Can you work these out from the model? Positions are in its coordinate system, mm. A direction names the side the tool comes from. Give positions to 0.01 mm unless a question says otherwise; leave off trailing zeros. Loops run counter-clockwise (first coordinate to the right, second up) from the corner with the lowest first, then second, coordinate; pieces in that order, holes last.
Solid Edge part; units mm, degrees
sketch "Sketch1" plane through (0, 0, 0) normal (1, 0, 0) x (0, 1, 0)
  circle A0 centre (0, 0) radius 2.5
extrude "Protrusion1" add sketch "Sketch1" along normal mid plane 40
sketch "Sketch2" plane through (0, 0, 0) normal (0, -1, 0) x (1, 0, 0)
  line L0 (30, 0) -> (30, 20)
  line L1 (30, -10) -> (30, 0)
  line L2 (20, -10) -> (30, -10)
  line L3 (20, 20) -> (20, -10)
  line L4 (20, 20) -> (-20, 20)
  line L5 (-20, -10) -> (-20, 20)
  line L6 (-30, -10) -> (-20, -10)
  line L7 (-30, 0) -> (-30, -10)
  line L8 (-30, 20) -> (-30, 0)
  line L9 (-30, 30) -> (-30, 20)
  line L10 (30, 30) -> (-30, 30)
  line L11 (30, 20) -> (30, 30)
extrude "ExtrudedProtrusion_2" add sketch "Sketch2" along normal mid plane 10
(1) Suppose I cut it at C-C on x = -14. List the corners of the cut face in (y, z) for me, plus the area to 3 significant figures.
Returned:
outline: (-5, 20) - (5, 20) - (5, 30) - (-5, 30) - close; circle Ø5 at (0, 0)
area: 120 mm2
(2) Will these pins go through, and if not, where does the flat tip stop? P1, Ø2, axis at x = -7, z = 18.5, coming from the -Y side; P2, Ø1, axis at x = -3, y = 2, coming from the -Z side.
Returned:
P1: passes through
P2: stops at z = -2
(3) Which directions (+Z, -Z, +X, -X, +Y, -Y) give clear straight access to the entire face, cutting with the end or side of a thin tool? Please do faces 5 (the flat face through (0, 0, 30)), 6 (the flat face through (0, 0, 20)).
Returned:
face 5: +Z, +X, -X, +Y, -Y
face 6: +Y, -Y
(4) Suppose I cut it at A-A on z = 6.5. List the corners of the cut face in (x, y) for me.
Returned:
outline: (-30, -5) - (-20, -5) - (-20, 5) - (-30, 5) - close; (20, -5) - (30, -5) - (30, 5) - (20, 5) - close
(5) Suppose I cut it at D-D on y = -3.75. List the corners of the cut face in (x, z) for me.
Returned:
outline: (-30, -10) - (-20, -10) - (-20, 20) - (20, 20) - (20, -10) - (30, -10) - (30, 30) - (-30, 30) - close
(6) Please list where these lines run through material, in increasing order: probe 1 along X at (y, z) = (0, 13); probe 2 along Z at (x, y) = (18, 0.25); probe 3 along Z at (x, y) = (-16.5, -3).
Returned:
probe 1: x = -30 to -20, 20 to 30
probe 2: z = -2.49 to 2.49, 20 to 30
probe 3: z = 20 to 30
(7) Thinking about a two-plate mould opening in X: for faces 1 (the flat face through (30, 0, 10)), 2 (the cylindrical face through (0.28, -0.54, -2.44)), 3 (the flat face through (-30, 0, 10)), 4 (the flat face through (-25, 0, -10)), which applies, pulls with the +X half, pulls with the -X half, needs draft (parallel to the pull), parting line crosses it, or undercut?
Returned:
face 1: pulls with the +X half
face 2: undercut
face 3: pulls with the -X half
face 4: needs draft
(8) Suppose I cut it at B-B on y = 0. List the corners of the cut face in (x, z) for me.
Returned:
outline: (-30, -10) - (-20, -10) - (-20, -2.5) - (20, -2.5) - (20, -10) - (30, -10) - (30, 30) - (-30, 30) - close; hole (-20, 2.5) - (20, 2.5) - (20, 20) - (-20, 20) - close
